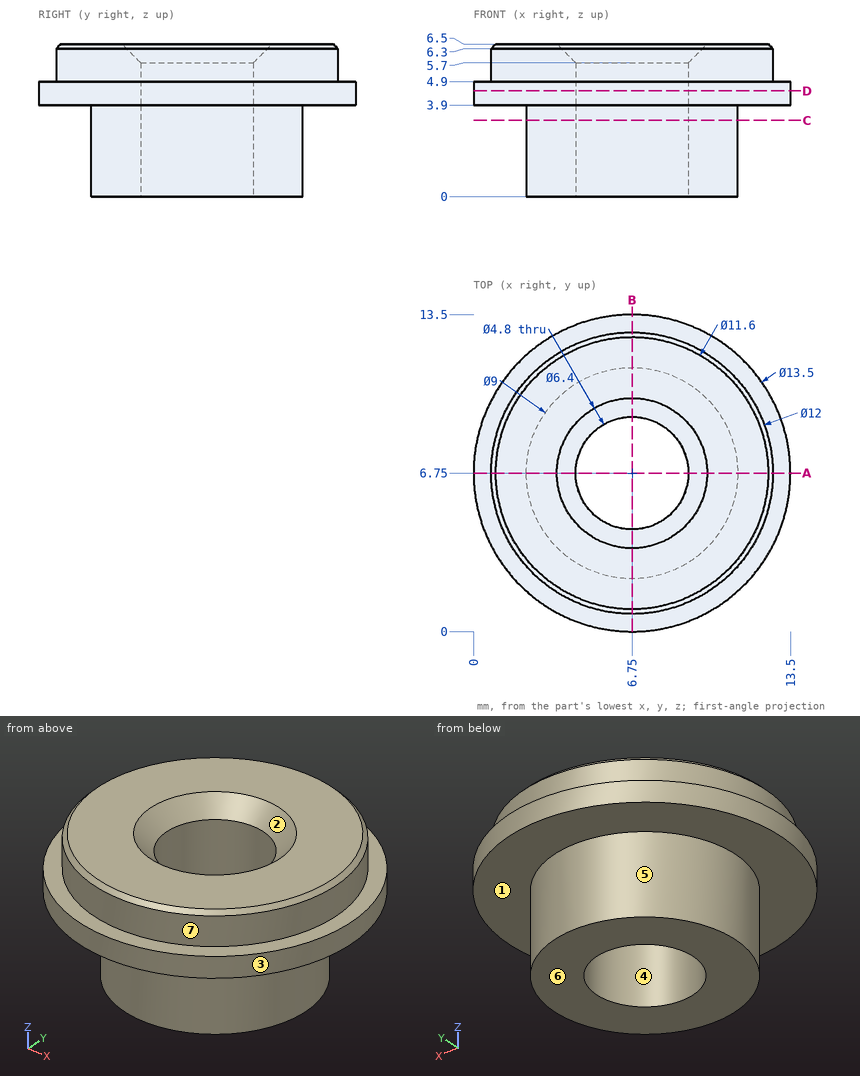
Geometry: see drawing. Coordinates: mm, zero at the bounding-box minimum. A direction names the side the tool comes from. Round coordinates to 2 decimals unless told otherwise and drop trailing zeros. Write each loop counter-clockwise with the first axis right and the second up, starting at its lowest first coordinate (ties: lowest second). Pieces come first, ordered by that corner, then holes.
1) Cut plane D-D (z = 4.5). Return the cut outline in (x, y).
2) Cut plane A-A (y = 6.75). Return the cut outline in (x, z), then the cut area to 3 significant figures.
3) Reachability of the marked faces 5, 6 and 7 from +Z, -Z, +X, -X, +Y, -Y: full face, straight path, thin tool, end or side. Return the list, or none.
4) Contact query for flat-ended pins moving along their axis: P1, Ø2, axis at x = 2, z = 1.5, coming from the +Y side; P2, Ø1.5, axis at x = 9.5, z = 5.5, coming from the -Y side; P3, Ø1.5, axis at x = 5.5, y = 7, coming from the +Z side. Output: stop coordinate, or through.
5) Ray query, L1, parallel to Y at x = 6.75, z = 4.2; L2, parallel to Z at x = 11.5, y = 7.25; L3, parallel to Y at x = 6.75, z = 1.3. Return the intervals inside material, ascending.
6) Cut plane C-C (z = 3.25). Return the cut outline in (x, y).
7) Draft query along X for the marked faces 1, 2, 3 and 4. Return one class per face: pulls with the +X half, pulls with the -X half, needs draft (parallel to the pull), parting line crosses it, or undercut.
Geometry says:
1. outline: circle Ø13.5 at (6.75, 6.75); hole circle Ø4.8 at (6.75, 6.75)
2. outline: (0, 3.9) - (2.25, 3.9) - (2.25, 0) - (4.35, 0) - (4.35, 5.7) - (3.55, 6.5) - (0.95, 6.5) - (0.75, 6.3) - (0.75, 4.9) - (0, 4.9) - close; (9.15, 0) - (11.25, 0) - (11.25, 3.9) - (13.5, 3.9) - (13.5, 4.9) - (12.75, 4.9) - (12.75, 6.3) - (12.55, 6.5) - (9.95, 6.5) - (9.15, 5.7) - close
2. area: 35.9 mm2
3. face 5: -Z
3. face 6: -Z, +X, -X, +Y, -Y
3. face 7: +Z
4. P1: stops at y = 9.24
4. P2: stops at y = 0.4
4. P3: passes through
5. L1: y = 0 to 4.35, 9.15 to 13.5
5. L2: z = 3.9 to 6.5
5. L3: y = 2.25 to 4.35, 9.15 to 11.25
6. outline: circle Ø9 at (6.75, 6.75); hole circle Ø4.8 at (6.75, 6.75)
7. face 1: needs draft
7. face 2: undercut
7. face 3: parting line crosses it
7. face 4: undercut
